```python
from build123d import *

# Parameters (mm, degrees)
BOSS_EXTRUDE1_DEPTH = 45.24375
SKETCH2_R           = 3.4925
BOSS_EXTRUDE2_DEPTH = 1.5875


with BuildPart() as part:
    # Sketch1 → Boss-Extrude1 (new body, symmetric)
    with BuildSketch(Plane(origin=(0, 0, 0), x_dir=(0, 0, -1), z_dir=(1, 0, 0))):
        with BuildLine():
            ThreePointArc((-26.121491242, 15.08125), (7.806629448, 29.134737735), (30.1625, 0))
            Line((30.1625, 0), (31.75, 0))
            ThreePointArc((31.75, 0), (8.217504682, 30.668144985), (-27.49630657, 15.875))
            Line((-27.49630657, 15.875), (-26.121491242, 15.08125))
        make_face()
    extrude(amount=BOSS_EXTRUDE1_DEPTH, both=True)

    # Sketch2 → Boss-Extrude2 (add)
    with BuildSketch(Plane(origin=(45.24375, 0, 0), x_dir=(0, 0, -1), z_dir=(1, 0, 0))):
        with BuildLine():
            Line((-19.05, 0), (-3.4925, 0))
            ThreePointArc((-3.4925, 0), (0, 3.4925), (3.4925, 0))
            Line((3.4925, 0), (19.05, 0))
            ThreePointArc((19.05, 0), (25.4, -6.35), (31.75, 0))
            ThreePointArc((31.75, 0), (0, 31.75), (-31.75, 0))
            ThreePointArc((-31.75, 0), (-25.4, -6.35), (-19.05, 0))
        make_face()
        with Locations((-25.4, 0)):
            Circle(SKETCH2_R, mode=Mode.SUBTRACT)
        with Locations((25.4, 0)):
            Circle(SKETCH2_R, mode=Mode.SUBTRACT)
    boss_extrude2 = extrude(amount=BOSS_EXTRUDE2_DEPTH)

    # Mirror1: Boss-Extrude2 across plane
    add(boss_extrude2.mirror(Plane(origin=(0, 0, 0), x_dir=(0, 0, 1), z_dir=(1, 0, 0))))


solid = part.part
```
Design review of the part built by this model. Coordinates are the model's own, in mm. A direction names the side the tool comes from. Coordinates: 2 decimals unless noted, no trailing zeros. Loops run counter-clockwise (first coordinate to the right, second up) from the corner with the lowest first, then second, coordinate; pieces in that order, holes last.
Q1. We need section C-C on z = -25.4. State the section outline as (x, y) points.
Reported:
outline: (-46.83, -6.35) - (-45.24, -6.35) - (-45.24, -3.49) - (-46.83, -3.49) - close; (-46.83, 3.49) - (-45.24, 3.49) - (-45.24, 16.27) - (45.24, 16.27) - (45.24, 3.49) - (46.83, 3.49) - (46.83, 19.05) - (-46.83, 19.05) - close; (45.24, -6.35) - (46.83, -6.35) - (46.83, -3.49) - (45.24, -3.49) - close
Q2. The part is to be moulded in two halves that separate along Y. For faces 3 (the face through (45.244, 12, 0)), 4 (the face through (-46.03, -6.35, 25.54)), 5 (the face through (-46.03, 0.15, 28.89)), say which applies: +Y half, -Y half, draft (parallel to the pull), parting line (faces both ways), or undercut.
Reported:
face 3: draft
face 4: -Y half
face 5: undercut
Q3. We need section A-A on z = 0. State the section outline as (x, y) points.
Reported:
outline: (-46.83, 3.49) - (-45.24, 3.49) - (-45.24, 30.16) - (45.24, 30.16) - (45.24, 3.49) - (46.83, 3.49) - (46.83, 31.75) - (-46.83, 31.75) - close
Q4. For pin 1 (1 mm diameter, centred on x = -18.5, z = 12.5, fed in from -Y); pin 2 (6 mm diameter, centred on x = 30, y = 1, fed in from +Z); pin 3 (1 mm diameter, centred on x = 30, z = -24, fed in from +Y); pin 4 (9 mm diameter, centred on y = 0, z = -25.4, fed in from +X), all flat-tipped, find the tip position at first contact; note any pin that passes through.
Reported:
pin 1: stops at y = 27.22
pin 2: stops at z = -29.9
pin 3: stops at y = 21.35
pin 4: stops at x = 46.83
Q5. We need section B-B on y = 29. State the section outline as (x, z) points, and give its area (3 significant figures).
Reported:
outline: (-46.83, -12.93) - (46.83, -12.93) - (46.83, 12.93) - (-46.83, 12.93) - close; hole (-45.24, -8.29) - (45.24, -8.29) - (45.24, 8.29) - (-45.24, 8.29) - close
area: 920 mm2
Q6. Tool access review of faces 1 (the face through (-45.244, 12, 0)), 2 (the face through (-46.831, 13, 0)): name each direction out of +Z, -Z, +X, -X, +Y, -Y from which nothing blocks a thin tool from reaching the whole face with its end or side.
Reported:
face 1: -Y
face 2: +Z, -Z, -X, +Y, -Y
Q7. To check wall thickness, follow line 1 (X direction, y = 1, z = -7.5); line 2 (Y direction, x = 46.45, z = 25.4); line 3 (Y direction, x = 0, z = -1). State the ranges of each line that lie inside material, in increasing order.
Reported:
line 1: x = -46.83 to -45.24, 45.24 to 46.83
line 2: y = -6.35 to -3.49, 3.49 to 19.05
line 3: y = 30.15 to 31.73
